The listing builds one solid part. Answer for the finished solid, in the listing's coordinates (mm). Round coordinates to 2 decimals unless told otherwise and drop trailing zeros. Loops run counter-clockwise (first coordinate to the right, second up) from the corner with the lowest first, then second, coordinate; pieces in that order, holes last. Notation, with made-up numbers: (-4.5, 49.25) -> (43.5, 49.25) arc R15 cw to (43.5, 72.25) -> close; hole circle Ø1 at (56, 74). An arc over 180 degrees is marked (long way). Write each question's results on one line, items separated by ' | '. Start each with the question number.
(1) The part is cut by section D-D (x = 58.5). Determine the outline of the cut face in (y, z), plus the area to 4 significant figures.
(2) Straight lines are drawn through the part: probe 1 along Y at (x, z) = (58.5, 2.8); probe 2 along X at (y, z) = (16, 3.9); probe 3 along X at (y, z) = (-28, 3.25). For each, find the intervals that lie inside material, in ascending order.
(3) The part is cut by section A-A (y = -31.5). Determine the outline of the cut face in (x, z), plus the area to 4 significant figures.
(4) The part is cut by section C-C (z = 1.15). Count the separate pieces of the cut face and the enclosed holes in it, plus the area to 3 significant figures.
(5) The part is cut by section B-B (x = 26). Determine the outline of the cut face in (y, z).
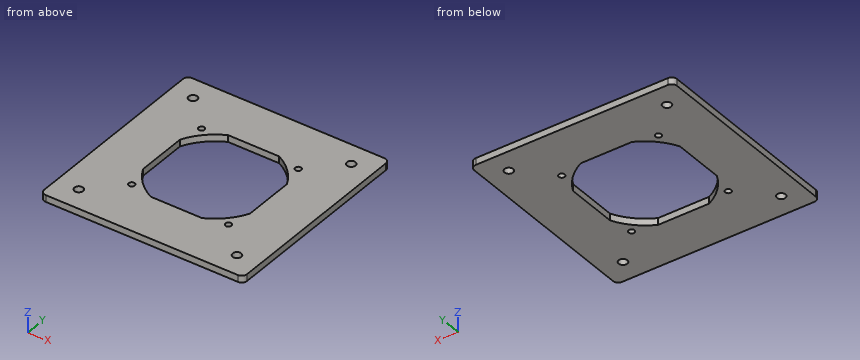
Autodesk Inventor part; units mm, degrees
ref_plane "YZ Plane" through (0, 0, 0) normal (1, 0, 0) x (0, 1, 0)
ref_plane "XZ Plane" through (0, 0, 0) normal (0, 1, 0) x (-1, 0, 0)
ref_plane "XY Plane" through (0, 0, 0) normal (0, 0, 1) x (1, 0, 0)
sketch "Boceto1" plane through (0, 0, 0) normal (0, 0, 1) x (1, 0, 0)
  line L0 (71, 32.2855) -> (-71, 32.2855)
  line L1 (-75, 28.2855) -> (-75, -113.7145)
  line L2 (-71, -117.7145) -> (71, -117.7145)
  line L3 (75, -113.7145) -> (75, 28.2855)
  line L4 (75, 32.2855) -> (-75, -117.7145) construction
  line L5 (-75, 32.2855) -> (75, -117.7145) construction
  circle A0 centre (35.75, -6.9645) radius 2.2
  circle A1 centre (35.75, -78.4645) radius 2.2
  circle A2 centre (-35.75, -78.4645) radius 2.2
  circle A3 centre (-35.75, -6.9645) radius 2.2
  arc A4 (39.55, -23.817) -> (18.8975, -3.1645) centre (0, -42.7145) ccw
  arc A5 (18.8975, -82.2645) -> (39.55, -61.612) centre (0, -42.7145) ccw
  arc A6 (-39.55, -61.612) -> (-18.8975, -82.2645) centre (0, -42.7145) ccw
  arc A7 (-18.8975, -3.1645) -> (-39.55, -23.817) centre (0, -42.7145) ccw
  line L6 (18.8975, -3.1645) -> (-18.8975, -3.1645)
  line L7 (39.55, -23.817) -> (39.55, -61.612)
  line L8 (18.8975, -82.2645) -> (-18.8975, -82.2645)
  line L9 (-39.55, -61.612) -> (-39.55, -23.817)
  line L10 (71, -117.7145) -> (42, -117.7145)
  line L11 (75, -84.7145) -> (75, -113.7145)
  line L12 (71, 32.2855) -> (42, 32.2855)
  line L13 (75, -0.7145) -> (75, 28.2855)
  line L14 (-71, 32.2855) -> (-42, 32.2855)
  line L15 (-75, -0.7145) -> (-75, 28.2855)
  line L16 (-71, -117.7145) -> (-42, -117.7145)
  line L17 (-75, -84.7145) -> (-75, -113.7145)
  line L18 (42, 32.2855) -> (75, -0.7145) construction
  line L19 (75, -84.7145) -> (42, -117.7145) construction
  line L20 (-75, -84.7145) -> (-42, -117.7145) construction
  line L21 (-42, 32.2855) -> (-75, -0.7145) construction
  circle A8 centre (-58.5, 15.7855) radius 3.175
  circle A9 centre (-58.5, -101.2145) radius 3.175
  circle A10 centre (58.5, 15.7855) radius 3.175
  circle A11 centre (58.5, -101.2145) radius 3.175
  arc A12 (75, 28.2855) -> (71, 32.2855) centre (71, 28.2855) ccw
  arc A13 (71, -117.7145) -> (75, -113.7145) centre (71, -113.7145) ccw
  arc A14 (-75, -113.7145) -> (-71, -117.7145) centre (-71, -113.7145) ccw
  arc A15 (-71, 32.2855) -> (-75, 28.2855) centre (-71, 28.2855) ccw
  arc A16 (18.8975, -82.2645) -> (39.55, -61.612) centre (0, -42.7145) ccw
  arc A17 (-39.55, -61.612) -> (-18.8975, -82.2645) centre (0, -42.7145) ccw
  arc A18 (39.55, -23.817) -> (18.8975, -3.1645) centre (0, -42.7145) ccw
  arc A19 (-18.8975, -3.1645) -> (-39.55, -23.817) centre (0, -42.7145) ccw
  point P0 (0, 0)
  dimension "d10" = 6.35
  dimension "d11" = 6.35
  dimension "d12" = 6.35
  dimension "d13" = 6.35
  dimension "d14" = 4
extrude "Extrusión1" add sketch "Boceto1" along normal blind 5
properties part number "TablaSoporte1" material "Madera (abedul)"
Checked values:
1) outline: (-117.71, 0) -> (-104.39, 0) -> (-104.39, 5) -> (-117.71, 5) -> close; (-98.04, 0) -> (12.61, 0) -> (12.61, 5) -> (-98.04, 5) -> close; (18.96, 0) -> (32.29, 0) -> (32.29, 5) -> (18.96, 5) -> close | area: 686.5 mm2
2) probe 1: y = -117.71 to -104.39, -98.04 to 12.61, 18.96 to 32.29 | probe 2: x = -75 to -61.67, -55.33 to 55.33, 61.67 to 75 | probe 3: x = -75 to -39.55, 39.55 to 75
3) outline: (-75, 0) -> (-39.55, 0) -> (-39.55, 5) -> (-75, 5) -> close; (39.55, 0) -> (75, 0) -> (75, 5) -> (39.55, 5) -> close | area: 354.5 mm2
4) separate pieces: 1 | enclosed holes: 9 | area: 16,700 mm2
5) outline: (-117.71, 0) -> (-78, 0) -> (-78, 5) -> (-117.71, 5) -> close; (-7.43, 0) -> (32.29, 0) -> (32.29, 5) -> (-7.43, 5) -> close
